Source: CAD feature listing. Evaluate the final solid. Frame: model axes, mm. A direction names the side the tool comes from. Round coordinates to 2 decimals unless told otherwise and drop trailing zeros. Order: outer loops, then holes, each group sorted by start corner. A loop starts at its lowest first (then second) coordinate and runs counter-clockwise, first axis right, second up. Notation, with made-up numbers: M 76.5,-8 L 129.5,-8 A12 ccw 129.5,10 Z; hole C 84,66 d2. An arc over 180 degrees is marked long. Use one line per item in the form item = value. Start each with the question number.
Q1. Section D-D (z = -12). Return the cut outline in (x, y).
Q2. Pull-direction query (Z, two-part tool) for faces 4 (the cylindrical face through (0.252, 7.144, 22.033)), 5 (the flat face through (18, 3, 4)), 6 (the cylindrical face through (0.147, -5.462, -12.846)); classes: pulls with the +Z half, pulls with the -Z half, needs draft (parallel to the pull), parting line crosses it, or undercut.
Q3. Reachability of faces 1 (the flat face through (0, -2, -18.494)), 2 (the flat face through (-10.5, -3, -15)), 3 (the flat face through (0, -2, -11.194)) from +Z, -Z, +X, -X, +Y, -Y: full face, straight path, thin tool, end or side. Return the list, or none.
Q4. Section C-C (x = -15.5). Return the cut outline in (y, z).
Q5. Material intervals for probe 1 along Y at (x, z) = (-14.5, -10); probe 2 along Z at (x, y) = (7, -1.25); probe 3 along Y at (x, z) = (0.5, 22), sorted ascending.
Q6. Contact query for flat-ended pins moving along their axis: pin 1 (1 mm diameter, centred on x = -11, y = 3.5, fed in from -Z); pin 2 (6 mm diameter, centred on x = 7.5, y = -1.5, fed in from +Z); pin 3 (3 mm diameter, centred on y = -2, z = 13, fed in from +X); pin 4 (3.5 mm diameter, centred on x = 2, y = -2, fed in from -Z). Output: stop coordinate, or through.
Q7. Section A-A (x = -9). Return the cut outline in (y, z), plus the area to 3 significant figures.
Q8. Section B-B (y = -5.55). Return the cut outline in (x, z), plus the area to 3 significant figures.
from build123d import *

# Parameters (mm, degrees)
BOSS_EXTRUDE1_DEPTH = 18
SKETCH2_W           = 21
SKETCH2_H           = 7.3
BOSS_EXTRUDE2_DEPTH = 8
CUT_EXTRUDE1_DEPTH  = 29.5
SKETCH4_R           = 2
CUT_EXTRUDE2_DEPTH  = 29.5


with BuildPart() as part:
    # Sketch1 → Boss-Extrude1 (new body, symmetric)
    with BuildSketch(Plane(origin=(0, 0, 0), x_dir=(0, 0, -1), z_dir=(1, 0, 0))):
        with BuildLine():
            Line((-13.605837563, 0), (18.494162437, 0))
            ThreePointArc((18.494162437, 0), (16.991105843, 4.690546334), (12.494162437, 6.7))
            Line((12.494162437, 6.7), (-17.505837563, 6.7))
            ThreePointArc((-17.505837563, 6.7), (-22.095938325, 7.156985164), (-26.505837563, 8.51))
            ThreePointArc((-26.505837563, 8.51), (-21.332902013, 2.319144372), (-13.605837563, 0))
        make_face()
    extrude(amount=BOSS_EXTRUDE1_DEPTH, both=True)

    # Sketch2 → Boss-Extrude2 (add)
    with BuildSketch(Plane.XZ):
        with Locations((0, -14.844162437)):
            Rectangle(SKETCH2_W, SKETCH2_H)
    extrude(amount=BOSS_EXTRUDE2_DEPTH)

    # Sketch3 → Cut-Extrude1 (cut, through all)
    with BuildSketch(Plane.ZY.offset(10.5)):
        with BuildLine():
            Line((-18.494162437, -4.35), (-18.494162437, -8))
            Line((-18.494162437, -8), (-14.844162437, -8))
            ThreePointArc((-14.844162437, -8), (-17.425102188, -6.930939751), (-18.494162437, -4.35))
        make_face()
        with BuildLine():
            ThreePointArc((-11.194162437, -4.35), (-12.263222685, -6.930939751), (-14.844162437, -8))
            Line((-14.844162437, -8), (-11.194162437, -8))
            Line((-11.194162437, -8), (-11.194162437, -4.35))
        make_face()
    extrude(amount=-CUT_EXTRUDE1_DEPTH, mode=Mode.SUBTRACT)

    # Sketch4 → Cut-Extrude2 (cut, through all)
    with BuildSketch(Plane(origin=(10.5, 0, 0), x_dir=(0, 0, -1), z_dir=(1, 0, 0))):
        with Locations((14.844162437, -5.55)):
            Circle(SKETCH4_R)
    extrude(amount=-CUT_EXTRUDE2_DEPTH, mode=Mode.SUBTRACT)


solid = part.part
Results list:
q1.outline = M -18,0 L -10.5,0 L -10.5,-6.64 L 10.5,-6.64 L 10.5,0 L 18,0 L 18,6.7 L -18,6.7 Z
q2.face_4 = pulls with the -Z half
q2.face_5 = needs draft
q2.face_6 = undercut
q3.face_1 = -Z, +X, -X, -Y
q3.face_2 = +Z, -Z, -X, -Y
q3.face_3 = +Z, +X, -X, -Y
q4.outline = M 0,-18.49 A6.04 ccw 6.7,-12.49 L 6.7,17.51 A23.28 cw 8.51,26.51 A14.03 ccw 0,13.61 Z
q5.probe_1 = 0 to 6.7
q5.probe_2 = -18.49 to -11.19
q5.probe_3 = 2.79 to 7.14
q6.pin_1 = -18.06
q6.pin_2 = 19.92
q6.pin_3 = through
q6.pin_4 = -18.49
q7.outline = M -4.35,-18.49 L 0,-18.49 A6.04 ccw 6.7,-12.49 L 6.7,17.51 A23.28 cw 8.51,26.51 A14.03 ccw 0,13.61 L 0,-11.19 L -4.35,-11.19 A3.65 ccw Z; hole C -5.55,-14.84 d4
q7.area = 309 mm2
q8.outline = M -10.5,-18.29 L 10.5,-18.29 L 10.5,-16.84 L -10.5,-16.84 Z; M -10.5,-12.84 L 10.5,-12.84 L 10.5,-11.4 L -10.5,-11.4 Z
q8.area = 60.8 mm2
